Could you check a few things on this model? Use its own coordinates, in mm. Face numbers are marked on the shaded views. Round coordinates to 2 decimals unless told otherwise and drop trailing zeros. Write each loop counter-clockwise with the first axis right and the second up, starting at its lowest first coordinate (ties: lowest second). Pieces come first, ordered by that corner, then holes. Notation, with made-up numbers: (-14, 34) - (45, 34) arc R30 cw to (45, 56) - close; hole circle Ø2 at (-36.5, 61.25). An arc over 180 degrees is marked (long way). Put each result on its own line as item: value.
from build123d import *

# Parameters (mm, degrees)
F2_R     = 13.5
F2_R_2   = 11
F3_DEPTH = 30
F5_R     = 7
F6_DEPTH = 10


# Not quite as in the source:
# - a fillet or chamfer that OpenCascade refuses, or shapes differently, is made with other operations: its cross-section is extruded or revolved along the edge and cut away or added


with BuildPart() as f1:
    # F0 (on Front) → F1 (revolve)
    with BuildSketch(Plane.XZ):
        with BuildLine():
            Line((0, 30), (0, 0))
            Line((0, 0), (60, 0))
            Line((60, 0), (60, 20))
            ThreePointArc((60, 20), (57.0710678119, 27.0710678119), (50, 30))
            Line((50, 30), (0, 30))
        make_face()
    revolve(axis=Axis((0, 0, 15), (0, 0, 1)))

    # F2 (on face) → F3 (join)
    with BuildSketch(Plane.XY.offset(30)):
        with Locations((0, 25)):
            Circle(F2_R)
        with Locations((0, 25)):
            Circle(F2_R_2, mode=Mode.SUBTRACT)
    extrude(amount=F3_DEPTH)

    # F4: fillet of radius 4 on 1 edges, made by hand

    # F4_s1 → F4_t2 (revolve, cut)
    with BuildSketch(Plane.XZ.offset(-25)):
        with BuildLine():
            ThreePointArc((13.5, 56.2919007565), (12.8166247904, 58.527968734), (11, 60))
            Line((11, 60), (13.5, 60))
            Line((13.5, 60), (13.5, 56.2919007565))
        make_face()
    revolve(axis=Axis((0, 25, 60), (0, 0, 1)), mode=Mode.SUBTRACT)

    # F5 (on face) → F6 (cut)
    with BuildSketch(Plane.XY.offset(30)):
        with Locations((0, -25)):
            Circle(F5_R)
    extrude(amount=-F6_DEPTH, mode=Mode.SUBTRACT)


solid = f1.part
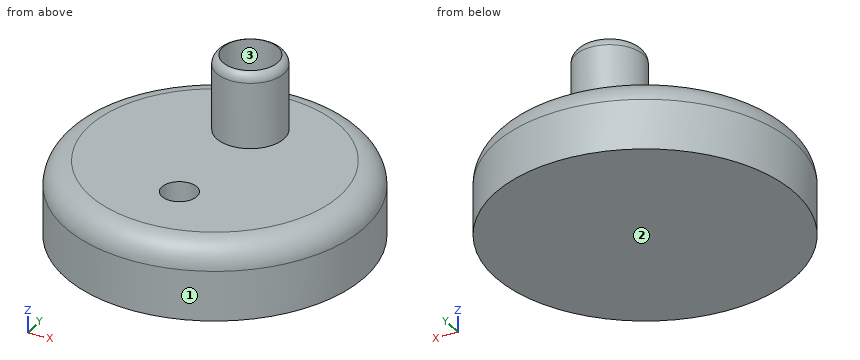
(1) Please list where these lines run through material, in increasing order: probe 1 along Y at (x, z) = (0, 42); probe 2 along Z at (x, y) = (37.5, 24); probe 3 along X at (y, z) = (21, 38). Write a range as from..to.
Values found:
probe 1: y = 11.5..14, 36..38.5
probe 2: z = 0..30
probe 3: x = -12.89..-10.25, 10.25..12.89
(2) I'm going to push flat-ended pins straight in: pin 1 (6.5 mm diameter, centred on x = -0.5, y = 23.5, fed in from +Z); pin 2 (3 mm diameter, centred on y = 24.5, z = 37.5, fed in from +X); pin 3 (4 mm diameter, centred on x = 2.5, y = -22, fed in from +Z). Where does each tip first touch, or does it pass through?
Values found:
pin 1: stops at z = 30
pin 2: stops at x = 13.5
pin 3: stops at z = 20
(3) Imagine slicing it at B-B, the plane z = 33. List the corners of the cut face in (x, y) for me.
Values found:
outline: circle Ø27 at (0, 25); hole circle Ø22 at (0, 25)
(4) If we mould it in two halves opening along Y, with no side actions, what happens to the marked faces 1, 2 and 3? For each: pulls with the +Y half, pulls with the -Y half, needs draft (parallel to the pull), parting line crosses it, or undercut.
Values found:
face 1: parting line crosses it
face 2: needs draft
face 3: undercut
(5) Imagine slicing it at A-A, the plane x = 0. List the corners of the cut face in (y, z) for me, then the cut area to 3 significant figures.
Values found:
outline: (-60, 0) - (60, 0) - (60, 20) arc R10 ccw to (50, 30) - (38.5, 30) - (38.5, 56.29) arc R4 ccw to (36, 60) - (36, 30) - (14, 30) - (14, 60) arc R4 ccw to (11.5, 56.29) - (11.5, 30) - (-18, 30) - (-18, 20) - (-32, 20) - (-32, 30) - (-50, 30) arc R10 ccw to (-60, 20) - close
area: 3,560 mm^2
